Work out the finished part from the listing and answer in its coordinate system (mm). A direction names the side the tool comes from. Coordinates: 2 decimals unless noted, no trailing zeros. Loops run counter-clockwise (first coordinate to the right, second up) from the corner with the lowest first, then second, coordinate; pieces in that order, holes last. Notation, with made-up numbers: (-37.5, -6.5) -> (-5.5, -6.5) arc R32 cw to (-5.5, 23.5) -> close; hole circle Ø6 at (10, -18). An arc over 180 degrees is marked (long way). Use a Markdown table: item, result.
from build123d import *

# Parameters (mm, degrees)
SKETCH1_W           = 17.78
SKETCH1_H           = 17.78
BOSS_EXTRUDE1_DEPTH = 1.5
CUT_EXTRUDE1_REACH  = 51.33
SKETCH2_R           = 1.804631731
SKETCH2_R_2         = 0.534898854
SKETCH3_W           = 3
SKETCH3_H           = 3
BOSS_EXTRUDE2_DEPTH = 0.9


with BuildPart() as part:
    # Sketch1 → Boss-Extrude1 (new body)
    with BuildSketch(Plane(origin=(0, 0, 0), x_dir=(1, 0, 0), z_dir=(0, 1, 0))):
        with Locations((-20.939781645, -30.370993212)):
            Rectangle(SKETCH1_W, SKETCH1_H)
    extrude(amount=BOSS_EXTRUDE1_DEPTH)

    # Sketch2 → Cut-Extrude1 (cut, up to next)
    with BuildSketch(Plane(origin=(0, 1.5, 0), x_dir=(1, 0, 0), z_dir=(0, 1, 0)), mode=Mode.PRIVATE) as cut_extrude1_sk1:
        with Locations(Location((-27.262286101, -23.941508984, 0), (0, 0, 270))):
            Circle(SKETCH2_R)
    cut_extrude1_tool1 = extrude(cut_extrude1_sk1.sketch, amount=-CUT_EXTRUDE1_REACH, mode=Mode.PRIVATE) & part.part
    # Sketch2 → Cut-Extrude1 (cut, up to next)
    with BuildSketch(Plane(origin=(0, 1.5, 0), x_dir=(1, 0, 0), z_dir=(0, 1, 0)), mode=Mode.PRIVATE) as cut_extrude1_sk2:
        with Locations(Location((-27.262286101, -36.693497669, 0), (0, 0, 270))):
            Circle(SKETCH2_R)
    cut_extrude1_tool2 = extrude(cut_extrude1_sk2.sketch, amount=-CUT_EXTRUDE1_REACH, mode=Mode.PRIVATE) & part.part
    # Sketch2 → Cut-Extrude1 (cut, up to next)
    with BuildSketch(Plane(origin=(0, 1.5, 0), x_dir=(1, 0, 0), z_dir=(0, 1, 0)), mode=Mode.PRIVATE) as cut_extrude1_sk3:
        with Locations(Location((-13.226540167, -26.466231576, 0), (0, 0, 270))):
            Circle(SKETCH2_R_2)
    cut_extrude1_tool3 = extrude(cut_extrude1_sk3.sketch, amount=-CUT_EXTRUDE1_REACH, mode=Mode.PRIVATE) & part.part
    # Sketch2 → Cut-Extrude1 (cut, up to next)
    with BuildSketch(Plane(origin=(0, 1.5, 0), x_dir=(1, 0, 0), z_dir=(0, 1, 0)), mode=Mode.PRIVATE) as cut_extrude1_sk4:
        with Locations(Location((-13.226540167, -29.006231576, 0), (0, 0, 270))):
            Circle(SKETCH2_R_2)
    cut_extrude1_tool4 = extrude(cut_extrude1_sk4.sketch, amount=-CUT_EXTRUDE1_REACH, mode=Mode.PRIVATE) & part.part
    # Sketch2 → Cut-Extrude1 (cut, up to next)
    with BuildSketch(Plane(origin=(0, 1.5, 0), x_dir=(1, 0, 0), z_dir=(0, 1, 0)), mode=Mode.PRIVATE) as cut_extrude1_sk5:
        with Locations(Location((-13.226540167, -31.546231576, 0), (0, 0, 270))):
            Circle(SKETCH2_R_2)
    cut_extrude1_tool5 = extrude(cut_extrude1_sk5.sketch, amount=-CUT_EXTRUDE1_REACH, mode=Mode.PRIVATE) & part.part
    # Sketch2 → Cut-Extrude1 (cut, up to next)
    with BuildSketch(Plane(origin=(0, 1.5, 0), x_dir=(1, 0, 0), z_dir=(0, 1, 0)), mode=Mode.PRIVATE) as cut_extrude1_sk6:
        with Locations(Location((-13.226540167, -34.086231576, 0), (0, 0, 270))):
            Circle(SKETCH2_R_2)
    cut_extrude1_tool6 = extrude(cut_extrude1_sk6.sketch, amount=-CUT_EXTRUDE1_REACH, mode=Mode.PRIVATE) & part.part
    add(cut_extrude1_tool1.solids().sort_by_distance((-27.262286, 1.5, 23.941509))[0], mode=Mode.SUBTRACT)
    add(cut_extrude1_tool2.solids().sort_by_distance((-27.262286, 1.5, 36.693498))[0], mode=Mode.SUBTRACT)
    add(cut_extrude1_tool3.solids().sort_by_distance((-13.22654, 1.5, 26.466232))[0], mode=Mode.SUBTRACT)
    add(cut_extrude1_tool4.solids().sort_by_distance((-13.22654, 1.5, 29.006232))[0], mode=Mode.SUBTRACT)
    add(cut_extrude1_tool5.solids().sort_by_distance((-13.22654, 1.5, 31.546232))[0], mode=Mode.SUBTRACT)
    add(cut_extrude1_tool6.solids().sort_by_distance((-13.22654, 1.5, 34.086232))[0], mode=Mode.SUBTRACT)

    # Sketch3 → Boss-Extrude2 (add)
    with BuildSketch(Plane(origin=(0, 1.5, 0), x_dir=(1, 0, 0), z_dir=(0, 1, 0))):
        with Locations((-20.801462442, -30.247030068)):
            Rectangle(SKETCH3_W, SKETCH3_H)
    extrude(amount=BOSS_EXTRUDE2_DEPTH)


solid = part.part
Q1. Section B-B on x = -21.5 is taken. Determine the outline of the cut face in (y, z).
Solved:
| item | result |
|---|---|
| outline | (0, 21.48) -> (1.5, 21.48) -> (1.5, 28.75) -> (2.4, 28.75) -> (2.4, 31.75) -> (1.5, 31.75) -> (1.5, 39.26) -> (0, 39.26) -> close |
Q2. Section D-D on z = 30.5 is taken. Determine the outline of the cut face in (x, y).
Solved:
| item | result |
|---|---|
| outline | (-29.83, 0) -> (-12.05, 0) -> (-12.05, 1.5) -> (-19.3, 1.5) -> (-19.3, 2.4) -> (-22.3, 2.4) -> (-22.3, 1.5) -> (-29.83, 1.5) -> close |
Q3. Section C-C on y = 1.2 is taken. Determine the outline of the cut face in (x, z).
Solved:
| item | result |
|---|---|
| outline | (-29.83, 21.48) -> (-12.05, 21.48) -> (-12.05, 39.26) -> (-29.83, 39.26) -> close; hole circle Ø3.61 at (-27.26, 23.94); hole circle Ø3.61 at (-27.26, 36.69); hole circle Ø1.07 at (-13.23, 26.47); hole circle Ø1.07 at (-13.23, 29.01); hole circle Ø1.07 at (-13.23, 31.55); hole circle Ø1.07 at (-13.23, 34.09) |
Q4. Section A-A on z = 26.25 is taken. Determine the outline of the cut face in (x, y), and give its area (3 significant figures).
Solved:
| item | result |
|---|---|
| outline | (-29.83, 0) -> (-13.72, 0) -> (-13.72, 1.5) -> (-29.83, 1.5) -> close; (-12.74, 0) -> (-12.05, 0) -> (-12.05, 1.5) -> (-12.74, 1.5) -> close |
| area | 25.2 mm² |
Q5. Determine the mould class of faces 5 (the cylindrical face through (-13.2, 0.76, 33.55)), 6 (the flat face through (-21, 1, 39.261)), 7 (the flat face through (-19.301, 2, 30)), 8 (the flat face through (-21, 1, 21.481)) for opening direction Z: pulls with the +Z half, pulls with the -Z half, needs draft (parallel to the pull), parting line crosses it, or undercut.
Solved:
| item | result |
|---|---|
| face 5 | undercut |
| face 6 | pulls with the +Z half |
| face 7 | needs draft |
| face 8 | pulls with the -Z half |
Q6. Given pin 1 Ø1.2 at (x, z) = (-13.23, 29.01) entering from +Y; pin 2 Ø2 at (x, z) = (-27.26, 36.69) entering from +Y, each flat-ended and moving along its own axis, determine where each tip first touches the part or whether it passes through.
Solved:
| item | result |
|---|---|
| pin 1 | y = 1.5 |
| pin 2 | through |
Q7. For faces 1 (the flat face through (-21, 2, 31.747)), 2 (the flat face through (-21, 2, 28.747)), 3 (the flat face through (-22.301, 2, 30)), 4 (the flat face through (-12.05, 1, 30)), determine the directions among +Z, -Z, +X, -X, +Y, -Y from which every point of the face is accessible in a straight line to the end or side of a thin tool.
Solved:
| item | result |
|---|---|
| face 1 | +Z, +X, -X, +Y |
| face 2 | -Z, +X, -X, +Y |
| face 3 | +Z, -Z, -X, +Y |
| face 4 | +Z, -Z, +X, +Y, -Y |
Q8. Consider line 1 (X direction, y = 0.35, z = 24); line 2 (Z direction, x = -12.75, y = 0.95); line 3 (Y direction, x = -25.5, z = 30). Determine where each line is inside the solid, lowest interval first. Write a range as [from, to].
Solved:
| item | result |
|---|---|
| line 1 | [-29.83, -29.07], [-25.46, -12.05] |
| line 2 | [21.48, 26.22], [26.71, 28.76], [29.25, 31.3], [31.79, 33.84], [34.33, 39.26] |
| line 3 | [0, 1.5] |
